from build123d import *

# Parameters (mm, degrees)
EXTRUDE_DEPTH = 2.5
TUBE_R        = 5
TUBE_R_2      = 2.6
TUBE_DEPTH    = 10


with BuildPart() as extrude_body:
    # Sketch → Extrude (new body, symmetric)
    with BuildSketch(Plane.XZ):
        Polygon((-10, 77), (10, 0), (30, 0), (0, 77), align=None)
    extrude(amount=EXTRUDE_DEPTH, both=True)


with BuildPart() as fusion:
    # Tube → Tube (new body)
    with BuildSketch(Plane(origin=(0, 0, 80), x_dir=(0, 0, 1), z_dir=(-1, 0, 0))):
        Circle(TUBE_R)
        Circle(TUBE_R_2, mode=Mode.SUBTRACT)
    extrude(amount=TUBE_DEPTH)

    # Fusion: union Extrude body
    add(extrude_body.part)


solid = fusion.part
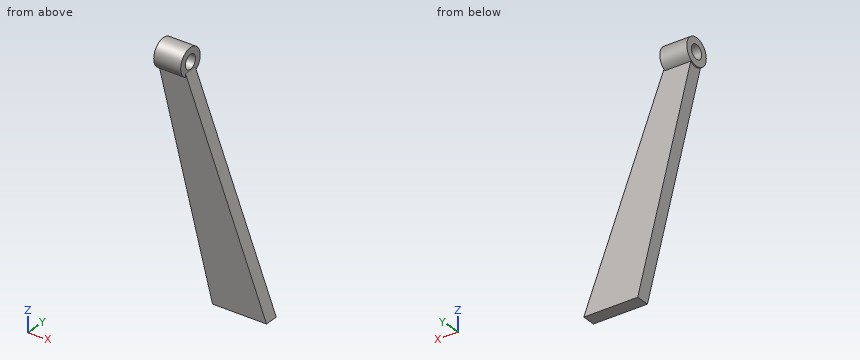
Can you work these out from the model? Positions are in its coordinate system, mm. Round coordinates to 2 decimals unless told otherwise and drop trailing zeros. Loops run counter-clockwise (first coordinate to the right, second up) from the corner with the lowest first, then second, coordinate; pieces in that order, holes last. Notation, with made-up numbers: (15.25, 21) - (50.25, 21) arc R8 ccw to (50.25, 28) - close; hole circle Ø10 at (34.5, 22.5). An arc over 180 degrees is marked (long way). Write item = value, one per line. Start each with the question number.
(1) If we section it at D-D (x = -1): Please give me the cut outline in (y, z), and give its area (3 significant figures).
(2) If we section it at C-C (y = 0): Please give me the cut outline in (x, z), and give its area (3 significant figures).
(3) If I drill on probe 1 along Y at (x, z) = (-3.25, 80); probe 2 along Y at (x, z) = (3.5, 39); probe 3 along X at (y, z) = (1, 5), over which ranges is the centre line in solid material (lowest first)? Write a range as [from, to].
(4) If we section it at B-B (z = 80): Please give me the cut outline in (x, y).
(5) If we section it at A-A (x = -5): Please give me the cut outline in (y, z).
(6) For P1, Ø1.5, axis at y = -2.5, z = 52.5, coming from the -X side; P2, Ø20, axis at x = 7.5, z = 48.5, coming from the +Y side; P3, Ø4, axis at y = 4, z = 29, coming from the -X side, each with a flat end and sliding along its axis, tell me the tip position at first contact or that it passes through.
Ans:
q1.outline = (-2.5, 42.35) - (2.5, 42.35) - (2.5, 75.67) arc R5 ccw (long way) to (-2.5, 75.67) - close; hole circle Ø5.2 at (0, 80)
q1.area = 222 mm²
q2.outline = (-10, 75) - (-9.48, 75) - (10, 0) - (30, 0) - (0, 77) - (0, 77.4) - (-10, 77.4) - close; (-10, 82.6) - (0, 82.6) - (0, 85) - (-10, 85) - close
q2.area = 1,180 mm²
q3.probe_1 = [-5, -2.6], [2.6, 5]
q3.probe_2 = [-2.5, 2.5]
q3.probe_3 = [8.7, 28.05]
q4.outline = (-10, -5) - (0, -5) - (0, -2.6) - (-10, -2.6) - close; (-10, 2.6) - (0, 2.6) - (0, 5) - (-10, 5) - close
q5.outline = (-2.5, 57.75) - (2.5, 57.75) - (2.5, 75.67) arc R5 ccw (long way) to (-2.5, 75.67) - close; hole circle Ø5.2 at (0, 80)
q6.P1 = -3.83
q6.P2 = 2.5
q6.P3 = 2.12
